```python
from build123d import *

# Parameters (mm, degrees)
SKETCH1_R              = 6.35
BOSS_EXTRUDE1_DEPTH    = 9.525
SKETCH2_R              = 2.413
CUT_EXTRUDE1_DEPTH     = 133.297838401
F_10_32_TAPPED_HOLE2_D = 4.0386
F_10_32_TAPPED_HOLE3_D = 4.0386
FILLET2_R              = 6.35
FILLET3_R              = 1.27
SKETCH15_R             = 1.5875
DOWEL_PIN_HOLE_DEPTH   = 100.600514289


with BuildPart() as part:
    # Sketch1 → Boss-Extrude1 (new body)
    with BuildSketch(Plane(origin=(0, 0, 0), x_dir=(0, 0, -1), z_dir=(1, 0, 0))):
        with BuildLine():
            Line((-85.0265, 88.20830847), (-85.0265, 100.90830847))
            Line((-85.0265, 100.90830847), (-19.05, 100.90830847))
            Line((-19.05, 100.90830847), (-6.703693037, 88.994416922))
            ThreePointArc((-6.703693037, 88.994416922), (-1.281815332, 76.848084565), (-5.804401761, 64.339033459))
            Line((-5.804401761, 64.339033459), (-15.875, 53.09280847))
            Line((-15.875, 53.09280847), (-15.875, 37.21780847))
            Line((-15.875, 37.21780847), (-31.75, 37.21780847))
            Line((-31.75, 37.21780847), (-31.75, 56.45830847))
            ThreePointArc((-31.75, 56.45830847), (-32.456751337, 58.164557133), (-34.163, 58.87130847))
            Line((-34.163, 58.87130847), (-34.2265, 58.87130847))
            Line((-34.2265, 58.87130847), (-34.2265, 88.20830847))
            Line((-34.2265, 88.20830847), (-85.0265, 88.20830847))
        make_face()
        with Locations(Location((-19.05, 76.2, 0), (0, 0, 180))):
            Circle(SKETCH1_R, mode=Mode.SUBTRACT)
    extrude(amount=BOSS_EXTRUDE1_DEPTH)

    # Sketch2 → Cut-Extrude1 (cut, through all)
    with BuildSketch(Plane(origin=(9.525, 0, 0), x_dir=(0, 0, -1), z_dir=(1, 0, 0))):
        with Locations((-35.932748663, 86.502059807)):
            Circle(SKETCH2_R)
    extrude(amount=-CUT_EXTRUDE1_DEPTH, mode=Mode.SUBTRACT)

    # #10-32 Tapped Hole2 (through all)
    with Locations(Plane(origin=(0, 88.20830847, 0), x_dir=(-1, 0, 0), z_dir=(0, -1, 0))):
        with Locations((-4.7625, -42.164), (-4.7625, -77.089)):
            Hole(F_10_32_TAPPED_HOLE2_D / 2)

    # #10-32 Tapped Hole3 (through all)
    with Locations(Plane.XY.offset(31.75)):
        with Locations((4.7625, 46.93330847)):
            Hole(F_10_32_TAPPED_HOLE3_D / 2)

    # Fillet2
    # the kernel refuses this fillet: 6.35 mm, written as the material it adds along each edge
    with BuildSketch(Plane(origin=(0, 53.09280847, 15.875), x_dir=(0, 0.7449717794882204, -0.6670959809248997), z_dir=(1, 0, 0))) as fillet2_piece_1:
        with BuildLine():
            CenterArc((FILLET2_R * 0.38229614299, -FILLET2_R), FILLET2_R, 90, 41.843324942)
            Line((-FILLET2_R * 0.284799837935, -FILLET2_R * 0.255028220512), (0, 0))
            Line((0, 0), (FILLET2_R * 0.38229614299, 0))
        make_face()
    extrude(amount=9.525)
    # the kernel refuses this fillet: 6.35 mm, written as the material it takes off along each edge
    with BuildSketch(Plane(origin=(-15.875, 100.90830847, 85.0265), x_dir=(0, -1, 0), z_dir=(1, 0, 0))) as fillet2_2_piece_1:
        with BuildLine():
            CenterArc((FILLET2_R, FILLET2_R), FILLET2_R, 180, 90)
            Line((0, FILLET2_R), (0, 0))
            Line((0, 0), (FILLET2_R, 0))
        make_face()
    extrude(amount=41.275, mode=Mode.SUBTRACT)
    with BuildSketch(Plane(origin=(-6.410510576, 100.90830847, 19.05), x_dir=(0, 0, 1), z_dir=(1, 0, 0))) as fillet2_2_piece_2:
        with BuildLine():
            CenterArc((FILLET2_R * 0.403811689842, FILLET2_R), FILLET2_R, 226.021135711, 43.978864289)
            Line((-FILLET2_R * 0.290581277715, FILLET2_R * 0.280403997644), (0, 0))
            Line((0, 0), (FILLET2_R * 0.403811689842, 0))
        make_face()
    extrude(amount=22.346021152, mode=Mode.SUBTRACT)
    with BuildSketch(Plane(origin=(-15.875, 37.21780847, 15.875), x_dir=(0, 0, 1), z_dir=(1, 0, 0))) as fillet2_2_piece_3:
        with BuildLine():
            CenterArc((FILLET2_R, -FILLET2_R), FILLET2_R, 90, 90)
            Line((0, -FILLET2_R), (0, 0))
            Line((0, 0), (FILLET2_R, 0))
        make_face()
    extrude(amount=41.275, mode=Mode.SUBTRACT)

    # Fillet3
    fillet3_edges = [part.edges().sort_by_distance(p)[0] for p in [
        (4.7625, 37.21780847, 31.75),
        (4.7625, 58.87130847, 34.2265),
        (4.7625, 88.20830847, 85.0265),
        (4.7625, 84.795811144, 34.2265),
        (4.7625, 88.20830847, 37.638997326),
    ]]
    fillet(fillet3_edges, radius=FILLET3_R)

    # Sketch15 → Dowel Pin hole (cut, through all)
    with BuildSketch(Plane.XZ.offset(-88.20830847)):
        with Locations(Location((4.7625, 59.6265, 0), (0, 0, 270))):
            Circle(SKETCH15_R)
    extrude(amount=-DOWEL_PIN_HOLE_DEPTH, mode=Mode.SUBTRACT)


solid = part.part
```
CAD build for the part. Positions are in the model's coordinates, mm. A direction names the side the tool comes from. Give positions to 0.01 mm unless a question says otherwise; leave off trailing zeros. Write each loop counter-clockwise with the first axis right and the second up, starting at its lowest first coordinate (ties: lowest second). Pieces come first, ordered by that corner, then holes. Notation, with made-up numbers: (-30, 82.5) -> (-4, 82.5) arc R36 ccw to (-4, 116.5) -> close; hole circle Ø10 at (-30.75, -13). An arc over 180 degrees is marked (long way). Write each question's results on one line, items separated by ' | '.
1. Two-plate mould, pull along Z, no slides. Class faces 4 (the flat face through (5, 100.908, 51)), 5 (the cylindrical face through (4.696, 57.84, 32.185)), 6 (the cylindrical face through (4.832, 94.469, 61.212)): pulls with the +Z half, pulls with the -Z half, needs draft (parallel to the pull), parting line crosses it, or undercut.
Geometry check:
face 4: needs draft | face 5: pulls with the +Z half | face 6: undercut
2. Wall check: probe 1 along Z at (x, y) = (5.75, 76.2); probe 2 along Y at (x, z) = (1.75, 63.5); probe 3 along Z at (x, y) = (9.25, 46) (3 decimals). Give the ranges that are in metal, low to high. Write a range as [from, to].
Geometry check:
probe 1: [1.27, 12.7], [25.4, 34.23] | probe 2: [88.21, 100.91] | probe 3: [15.875, 31.75]
3. Drop flat-ended pins along their axis: P1, Ø2.5, axis at x = 4.76, y = 46.93, coming from the +Z side; P2, Ø5, axis at x = 3.5, z = 65, coming from the -Y side; P3, Ø3, axis at x = 3.5, y = 61, coming from the +Z side; P4, Ø2, axis at x = 3, y = 45.5, coming from the -Z side (3 decimals). Give the stop position or say it passes through.
Geometry check:
P1: through | P2: y = 88.21 | P3: z = 34.23 | P4: z = 15.875
4. Cut at D-D, the plane y = 68. Write the cut outline in (x, z) (1 decimal), then the cut area to 3 significant figures.
Geometry check:
outline: (0, 3.3) -> (9.5, 3.3) -> (9.5, 34.2) -> (0, 34.2) -> close | area: 295 mm²
5. Cut at C-C, the plane z = 73. Write the cut outline in (x, y) (3 decimals), then the cut area to 3 significant figures.
Geometry check:
outline: (0, 88.208) -> (9.525, 88.208) -> (9.525, 100.908) -> (0, 100.908) -> close | area: 121 mm²
6. Cut at A-A, the plane z = 19.05. Give the number of separate pieces and of enclosed holes in the cut face, then the cut area to 3 significant figures.
Geometry check:
separate pieces: 2 | enclosed holes: 1 | area: 460 mm²
7. Cut at B-B, the plane y = 76.2. Write the cut outline in (x, z) (1 decimal), then the cut area to 3 significant figures.
Geometry check:
outline: (0, 1.3) -> (9.5, 1.3) -> (9.5, 12.7) -> (0, 12.7) -> close; (0, 25.4) -> (9.5, 25.4) -> (9.5, 34.2) -> (0, 34.2) -> close | area: 193 mm²
8. Which spindle directions (+Z, -Z, +X, -X, +Y, -Y) get a long thin tool onto all of the face, cutting with end or side? Do faces 1 (the flat face through (4.696, 94.132, 12.028)), 2 (the flat face through (5, 72, 34.226)), 3 (the flat face through (6, 49, 15.875)). Say none if no direction does.
Geometry check:
face 1: -Z, +X, -X, +Y | face 2: +Z, +X, -X, -Y | face 3: -Z, +X, -X, -Y
